The listing builds one solid part. Answer for the finished solid, in the listing's coordinates (mm). A direction names the side the tool comes from. Round coordinates to 2 decimals unless told otherwise and drop trailing zeros. Order: outer loops, then holes, each group sorted by start corner. A loop starts at its lowest first (then second) coordinate and runs counter-clockwise, first axis right, second up. Notation, with made-up numbers: (3.5, 68) -> (58.5, 68) arc R18 cw to (58.5, 91) -> close; hole circle Ø11 at (-4, 4). An arc over 180 degrees is marked (long way). Return JSON: item names as keys, results as strings. Group by question number.
(1) Consider line 1 (Z direction, x = -57.5, y = 155.5); line 2 (Y direction, x = -73, z = -4.25); line 3 (Y direction, x = -65, z = -0.75). Determine where each line is inside the solid, lowest interval first. Write a range as [from, to].
(2) Each of these flat-tipped pins is pushed along its axis until it touches: pin 1 (5 mm diameter, centred on x = -79.5, z = -6, fed in from +Y); pin 2 (8 mm diameter, centred on y = 168, z = 7.5, fed in from -X); pin 3 (3 mm diameter, centred on y = 21, z = 2, fed in from +X); pin 4 (3.5 mm diameter, centred on y = 172.5, z = -6, fed in from -X). Where does it stop, or does it pass through?
(3) The part is cut by section A-A (x = -72). Determine the outline of the cut face in (y, z), plus the area to 3 significant figures.
(4) Determine the mould class of faces 5 (the face through (-73, 188, 8.1)), 6 (the face through (-73, 158, 8)), 7 (the face through (-73, 178, 11.1)), 8 (the face through (-73, 177.8, 0)) for opening direction Z: +Z half, -Z half, draft (parallel to the pull), parting line (faces both ways), or undercut.
(5) Which of the six approach directions +Z, -Z, +X, -X, +Y, -Y give full straight-line access (tool end or side, diameter ignored) to faces 1 (the face through (-73, 188, -8.1)), 2 (the face through (-59, 173, -8)), 3 (the face through (-87, 173, 8)), 4 (the face through (-87, 173, -8))?
(6) The part is cut by section C-C (z = 0). Determine the outline of the cut face in (x, y), plus the area to 3 significant figures.
(7) The part is cut by section D-D (x = -109). Determine the outline of the cut face in (y, z), plus the area to 3 significant figures.
(8) The part is cut by section B-B (y = 170.5). Determine the outline of the cut face in (x, z).
from build123d import *

# Parameters (mm, degrees)
BOSS_EXTRUDE1_DEPTH = 4
BOSS_EXTRUDE2_START = 158
SKETCH2_W           = 28
SKETCH2_H           = 22.2
BOSS_EXTRUDE2_DEPTH = 19.8
BOSS_EXTRUDE3_START = 177.8
SKETCH3_W           = 28
SKETCH3_H           = 3
BOSS_EXTRUDE3_DEPTH = 20


with BuildPart() as part:
    # Sketch1 → Boss-Extrude1 (new, symmetric)
    with BuildSketch(Plane.XY):
        Polygon((-115, 0), (-45, 0), (-59, 177.8), (-87, 177.8), align=None)
    extrude(amount=BOSS_EXTRUDE1_DEPTH, both=True)

    # Sketch2 → Boss-Extrude2 (add)
    with BuildSketch(Plane(origin=(0, 0, 0), x_dir=(1, 0, 0), z_dir=(0, 1, 0)).offset(BOSS_EXTRUDE2_START)):
        with Locations((-73, 0)):
            Rectangle(SKETCH2_W, SKETCH2_H)
    extrude(amount=BOSS_EXTRUDE2_DEPTH)

    # Sketch3 → Boss-Extrude3 (add)
    with BuildSketch(Plane(origin=(0, 0, 0), x_dir=(1, 0, 0), z_dir=(0, 1, 0)).offset(BOSS_EXTRUDE3_START)):
        with Locations((-73, 9.6)):
            Rectangle(SKETCH3_W, SKETCH3_H)
        with Locations((-73, -9.6)):
            Rectangle(SKETCH3_W, SKETCH3_H)
    extrude(amount=BOSS_EXTRUDE3_DEPTH)


solid = part.part
Answer below:
{
 "1": {"line 1": "z = [-4, 4]", "line 2": "y = [158, 177.8]", "line 3": "y = [0, 177.8]"},
 "2": {"pin 1": "stops at y = 197.8", "pin 2": "stops at x = -88.85", "pin 3": "stops at x = -46.54", "pin 4": "stops at x = -87"},
 "3": {"outline": "(0, -4) -> (158, -4) -> (158, -11.1) -> (197.8, -11.1) -> (197.8, -8.1) -> (177.8, -8.1) -> (177.8, 8.1) -> (197.8, 8.1) -> (197.8, 11.1) -> (158, 11.1) -> (158, 4) -> (0, 4) -> close", "area": "1,820 mm²"},
 "4": {"face 5": "undercut", "face 6": "draft", "face 7": "+Z half", "face 8": "undercut"},
 "5": {"face 1": "+X, -X, +Y", "face 2": "-Z, +X, +Y, -Y", "face 3": "+Z, -X, +Y, -Y", "face 4": "-Z, -X, +Y, -Y"},
 "6": {"outline": "(-115, 0) -> (-45, 0) -> (-59, 177.8) -> (-87, 177.8) -> close", "area": "8,710 mm²"},
 "7": {"outline": "(0, -4) -> (38.1, -4) -> (38.1, 4) -> (0, 4) -> close", "area": "305 mm²"},
 "8": {"outline": "(-88.15, -4) -> (-87, -4) -> (-87, -11.1) -> (-59, -11.1) -> (-59, -4) -> (-58.43, -4) -> (-58.43, 4) -> (-59, 4) -> (-59, 11.1) -> (-87, 11.1) -> (-87, 4) -> (-88.15, 4) -> close"}
}
